from build123d import *

# Parameters (mm, degrees)
F0_R     = 3.175
F0_R_2   = 3.5
F1_DEPTH = 9


# Not quite as in the source:
# - ends of sketch curves that miss each other by under 0.0002 mm in the source are joined


with BuildPart() as f1:
    # F0 (on Top) → F1 (new body)
    with BuildSketch(Plane.XY):
        with BuildLine():
            Line((0, 25.675), (0, 37.5))
            Line((0, 37.5), (-31, 37.5))
            ThreePointArc((-31, 37.5), (-37.3639610307, 34.8639610307), (-40, 28.5))
            Line((-40, 28.5), (-40, 27.5))
            ThreePointArc((-40, 27.5), (-44.1005050634, 17.6005050634), (-54, 13.5))
            ThreePointArc((-54, 13.5), (-54.7071067812, 13.2071067812), (-55, 12.5))
            Line((-55, 12.5), (-55, 0))
            Line((-55, 0), (-46.175, 0))
            ThreePointArc((-46.175, 0), (-41, 5.175), (-35.825, 0))
            Line((-35.825, 0), (-25.675, 0))
            ThreePointArc((-25.675, 0), (-22.5, 3.175), (-19.325, 0))
            Line((-19.325, 0), (-11.5, 0))
            ThreePointArc((-11.5, 0), (-8.1317279836, 8.1317279836), (0, 11.5))
            Line((0, 11.5), (0, 19.325))
            ThreePointArc((0, 19.325), (-3.175, 22.5), (0, 25.675))
        make_face()
        with BuildLine():
            ThreePointArc((-30.5652871781, 5.0672249135), (-34.9739264655, 9.9119341078), (-41.3041070016, 11.5960130619))
            ThreePointArc((-41.3041070016, 11.5960130619), (-37.2403076286, 15.9572441931), (-34.6146149846, 21.3089299951))
            ThreePointArc((-34.6146149846, 21.3089299951), (-21.4024086548, 17.845567287), (-18.3122078194, 31.1500001161))
            Line((-18.3122078194, 31.1500001161), (-3.987873, 31.15))
            ThreePointArc((-3.987873, 31.15), (-9.3036595822, 24.5414561908), (-7.2431808946, 16.31437509))
            ThreePointArc((-7.2431808946, 16.31437509), (-12.6218560442, 12.6218560442), (-16.3143749324, 7.24318097))
            ThreePointArc((-16.3143749324, 7.24318097), (-23.9376990029, 9.4158720561), (-30.5652871781, 5.0672249135))
        make_face(mode=Mode.SUBTRACT)
        with Locations((-26.324893, 26)):
            Circle(F0_R, mode=Mode.SUBTRACT)
        with BuildLine():
            ThreePointArc((0, -11.5), (-8.1317279836, -8.1317279836), (-11.5, 0))
            Line((-11.5, 0), (-19.325, 0))
            ThreePointArc((-19.325, 0), (-22.5, -3.175), (-25.675, 0))
            Line((-25.675, 0), (-35.825, 0))
            ThreePointArc((-35.825, 0), (-41, -5.175), (-46.175, 0))
            Line((-46.175, 0), (-55, 0))
            Line((-55, 0), (-55, -12.5))
            ThreePointArc((-55, -12.5), (-54.7071067812, -13.2071067812), (-54, -13.5))
            ThreePointArc((-54, -13.5), (-44.1005050634, -17.6005050634), (-40, -27.5))
            Line((-40, -27.5), (-40, -28.5))
            ThreePointArc((-40, -28.5), (-37.3639610307, -34.8639610307), (-31, -37.5))
            Line((-31, -37.5), (0, -37.5))
            Line((0, -37.5), (0, -25.675))
            ThreePointArc((0, -25.675), (-3.175, -22.5), (0, -19.325))
            Line((0, -19.325), (0, -11.5))
        make_face()
        with Locations((-26.324893, -26)):
            Circle(F0_R, mode=Mode.SUBTRACT)
        with BuildLine():
            ThreePointArc((-34.6146149846, -21.3089299951), (-37.2403076286, -15.9572441931), (-41.304107024, -11.59601303))
            ThreePointArc((-41.304107024, -11.59601303), (-34.9739264655, -9.9119341078), (-30.5652871781, -5.0672249135))
            ThreePointArc((-30.5652871781, -5.0672249135), (-23.9376990029, -9.4158720561), (-16.31437509, -7.2431808946))
            ThreePointArc((-16.31437509, -7.2431808946), (-12.6218560442, -12.6218560442), (-7.24318097, -16.3143749324))
            ThreePointArc((-7.24318097, -16.3143749324), (-9.3036595822, -24.5414561908), (-3.9878728667, -31.1499997109))
            Line((-3.9878728667, -31.1499997109), (-18.312208, -31.15))
            ThreePointArc((-18.312208, -31.15), (-21.4024086548, -17.845567287), (-34.6146149846, -21.3089299951))
        make_face(mode=Mode.SUBTRACT)
        with BuildLine():
            Line((19.325, 0), (11.5, 0))
            ThreePointArc((11.5, 0), (8.1317279836, -8.1317279836), (0, -11.5))
            Line((0, -11.5), (0, -19.325))
            ThreePointArc((0, -19.325), (2.2450640303, -20.2549359697), (3.175, -22.5))
            ThreePointArc((3.175, -22.5), (2.2450640303, -24.7450640303), (0, -25.675))
            Line((0, -25.675), (0, -37.5))
            Line((0, -37.5), (31, -37.5))
            ThreePointArc((31, -37.5), (37.3639610307, -34.8639610307), (40, -28.5))
            Line((40, -28.5), (40, -27.5))
            ThreePointArc((40, -27.5), (44.1005050634, -17.6005050634), (54, -13.5))
            ThreePointArc((54, -13.5), (54.7071067812, -13.2071067812), (55, -12.5))
            Line((55, -12.5), (55, 0))
            Line((55, 0), (46.175, 0))
            ThreePointArc((46.175, 0), (41, -5.175), (35.825, 0))
            Line((35.825, 0), (25.675, 0))
            ThreePointArc((25.675, 0), (22.5, -3.175), (19.325, 0))
        make_face()
        with Locations((26.324893, -26)):
            Circle(F0_R, mode=Mode.SUBTRACT)
        with BuildLine():
            ThreePointArc((7.24318097, -16.3143749324), (12.6218560442, -12.6218560442), (16.3143749324, -7.24318097))
            ThreePointArc((16.3143749324, -7.24318097), (20.5869660419, -9.3309123924), (25.3363869117, -9.0928837168))
            ThreePointArc((25.3363869117, -9.0928837168), (25.3425465049, -12.93806398), (26.8204236463, -16.4878985664))
            ThreePointArc((26.8204236463, -16.4878985664), (18.0864944073, -21.2193710008), (18.3122078194, -31.1500001161))
            Line((18.3122078194, -31.1500001161), (3.987872, -31.15))
            ThreePointArc((3.987872, -31.15), (9.3036594849, -24.5414566343), (7.24318097, -16.3143749324))
        make_face(mode=Mode.SUBTRACT)
        with Locations((35, -11)):
            Circle(F0_R_2, mode=Mode.SUBTRACT)
        with BuildLine():
            Line((31, 37.5), (0, 37.5))
            Line((0, 37.5), (0, 25.675))
            ThreePointArc((0, 25.675), (2.2450640303, 24.7450640303), (3.175, 22.5))
            ThreePointArc((3.175, 22.5), (2.2450640303, 20.2549359697), (0, 19.325))
            Line((0, 19.325), (0, 11.5))
            ThreePointArc((0, 11.5), (8.1317279836, 8.1317279836), (11.5, 0))
            Line((11.5, 0), (19.325, 0))
            ThreePointArc((19.325, 0), (22.5, 3.175), (25.675, 0))
            Line((25.675, 0), (35.825, 0))
            ThreePointArc((35.825, 0), (41, 5.175), (46.175, 0))
            Line((46.175, 0), (55, 0))
            Line((55, 0), (55, 12.5))
            ThreePointArc((55, 12.5), (54.7071067812, 13.2071067812), (54, 13.5))
            ThreePointArc((54, 13.5), (44.1005050634, 17.6005050634), (40, 27.5))
            Line((40, 27.5), (40, 28.5))
            ThreePointArc((40, 28.5), (37.3639610307, 34.8639610307), (31, 37.5))
        make_face()
        with BuildLine():
            ThreePointArc((30.5652870625, 5.0672250393), (23.9376990029, 9.4158720561), (16.31437509, 7.2431808946))
            ThreePointArc((16.31437509, 7.2431808946), (12.6218560442, 12.6218560442), (7.24318097, 16.3143749324))
            ThreePointArc((7.24318097, 16.3143749324), (9.3036594849, 24.5414566343), (3.987872042, 31.1500000911))
            Line((3.987872042, 31.1500000911), (18.312208, 31.15))
            ThreePointArc((18.312208, 31.15), (21.4024086548, 17.845567287), (34.6146148363, 21.3089300926))
            ThreePointArc((34.6146148363, 21.3089300926), (37.2403076286, 15.9572441931), (41.304107024, 11.59601303))
            ThreePointArc((41.304107024, 11.59601303), (34.9739264655, 9.9119341078), (30.5652870625, 5.0672250393))
        make_face(mode=Mode.SUBTRACT)
        with Locations((26.324893, 26)):
            Circle(F0_R, mode=Mode.SUBTRACT)
    extrude(amount=F1_DEPTH)


solid = f1.part
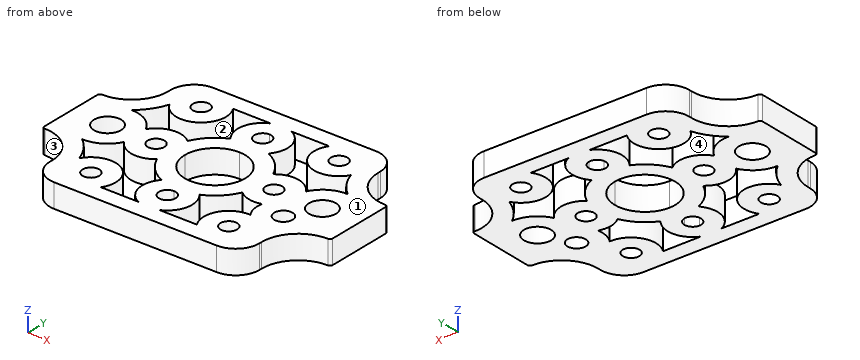
Geometry: final body of the model. Coordinates: model frame, mm. Face numbers are marked on the shaded views. Round coordinates to 2 decimals unless told otherwise and drop trailing zeros. Loops run counter-clockwise (first coordinate to the right, second up) from the corner with the lowest first, then second, coordinate; pieces in that order, holes last. Notation, with made-up numbers: M 83.5,70 L 93.5,70 A18 ccw 93.5,82 Z; hole C 7,45 d11. An arc over 180 degrees is marked long. One line per question, with ' | ' between items.
(1) Cut plane B-B on y = 24.5. Return the cut outline in (x, z).
Check result:
outline: M -40.33,0 L -29.12,0 L -29.12,9 L -40.33,9 Z; M -23.53,0 L -16.92,0 L -16.92,9 L -23.53,9 Z; M -9.31,0 L -2.47,0 L -2.47,9 L -9.31,9 Z; M 2.47,0 L 9.31,0 L 9.31,9 L 2.47,9 Z; M 16.92,0 L 23.53,0 L 23.53,9 L 16.92,9 Z; M 29.12,0 L 40.33,0 L 40.33,9 L 29.12,9 Z
(2) Cut plane A-A on x = -13. Return the cut outline in (y, z), plus the area to 3 significant figures.
Check result:
outline: M -37.5,0 L -31.15,0 L -31.15,9 L -37.5,9 Z; M -12.23,0 L 12.23,0 L 12.23,9 L -12.23,9 Z; M 31.15,0 L 37.5,0 L 37.5,9 L 31.15,9 Z | area: 334 mm2
(3) Pull-direction query (Y, two-part tool) for the marked faces 1, 2, 3 and 4; classes: +Y half, -Y half, draft (parallel to the pull), parting line (faces both ways), or undercut.
Check result:
face 1: draft | face 2: undercut | face 3: -Y half | face 4: undercut
(4) Material intervals for line 1 along X through (y, z) = (-27.5, 8.5); line 2 along Y through (x, z) = (-22.5, 5) (3 decimals); line 3 along Y through (x, z) = (8, 2.75), sorted ascending. Write a range as from..to.
Check result:
line 1: x = -40..-29.12, -23.53..-16.92, -8.11..8.11, 16.92..23.53, 29.12..40 | line 2: y = -37.5..-17.277, -9.525..-3.175, 3.175..9.525, 17.277..37.5 | line 3: y = -37.5..-31.15, -27.67..-17.33, -15.96..-8.26, 8.26..15.96, 17.33..27.67, 31.15..37.5
(5) Cut plane D-D on x = 20.5. Return the cut outline in (y, z), plus the area to 3 significant figures.
Check result:
outline: M -37.5,0 L -18.46,0 L -18.46,9 L -37.5,9 Z; M -9.31,0 L -2.47,0 L -2.47,9 L -9.31,9 Z; M 2.47,0 L 9.31,0 L 9.31,9 L 2.47,9 Z; M 18.46,0 L 37.5,0 L 37.5,9 L 18.46,9 Z | area: 466 mm2
(6) Cut plane C-C on z = 5.75. Give the number of separate pieces and of enclosed holes in the cut face, plus the area to 3 significant figures.
Check result:
separate pieces: 1 | enclosed holes: 16 | area: 4,680 mm2
(7) Contact query for flat-ended pins moving along their axis: P1, Ø0.8, axis at y = -28, z = 4.5, coming from the +X side; P2, Ø4, axis at x = -26.32, y = 26, coming from the +Z side; P3, Ø1.5, axis at y = 22, z = 2, coming from the -X side; P4, Ø0.8, axis at y = -28, z = 2.5, coming from the -X side. Output: stop coordinate, or through.
Check result:
P1: stops at x = 40 | P2: passes through | P3: stops at x = -41.47 | P4: stops at x = -40
